Geometry: see drawing. Coordinates: mm, zero at the bounding-box minimum. A direction names the side the tool comes from. Round coordinates to 2 decimals unless told otherwise and drop trailing zeros. Write each loop counter-clockwise with the first axis right and the second up, starting at its lowest first coordinate (ties: lowest second). Pieces come first, ordered by that corner, then holes.
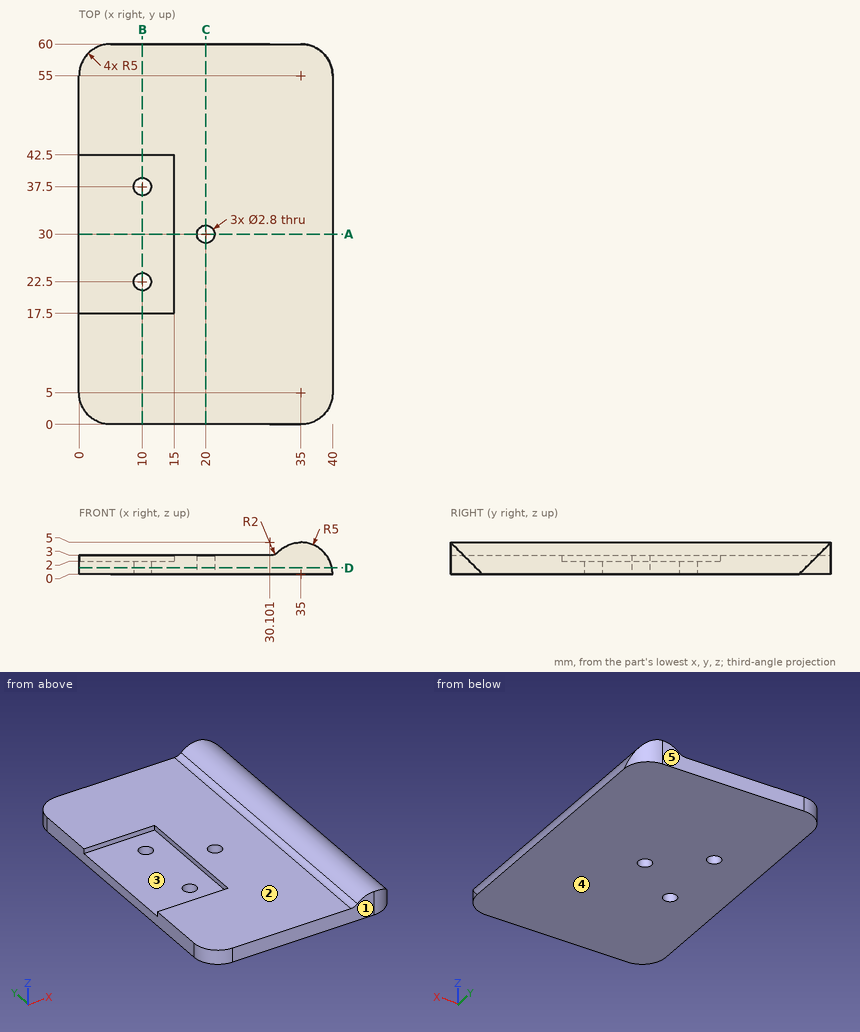
Q1. Set-up query: the marked faces 1 and 2. Return all of +Z, -Z, +X, -X, +Y, -Y with unobstructed straight access to the full face (end or side cutting, diameter ignored); none if empty.
Q2. Pin query (flat end, axial travel): P1, Ø2.5, axis at x = 20, y = 30, coming from the -Z side; P2, Ø8, axis at x = 16, y = 42.5, coming from the +Z side; P3, Ø0.8, axis at y = 28.5, z = 2.5, coming from the -X side; P4, Ø4.5, axis at x = 6.5, y = 27, coming from the +Z side. Return the tip coordinate at first contact, or that it passes through.
Q3. Section query A-A, the plane y = 30. Output: boundary loops of the cut face in (x, z).
Q4. Section query C-C, the plane x = 20. Output: boundary loops of the cut face in (y, z), and give its area (3 significant figures).
Q5. Mould query, pull axis Y, two halves, no side actions, for the marked faces 3, 4 and 5. Classes: pulls with the +Y half, pulls with the -Y half, needs draft (parallel to the pull), parting line crosses it, or undercut.
Q6. Line query: line 1 (Y direction, x = 10, z = 0.9); line 2 (Y direction, x = 20, z = 1.75); line 3 (Z direction, x = 20, y = 56). Output: solid intervals per line, ascending.
Q7. Section query D-D, the plane z = 1. Output: boundary loops of the cut face in (x, y).
Q8. Section query B-B, the plane x = 10. Output: boundary loops of the cut face in (y, z).
Filled in:
1. face 1: +Z, -Z, +X, -X, -Y
1. face 2: +Z, -X, +Y, -Y
2. P1: passes through
2. P2: stops at z = 3
2. P3: stops at x = 15
2. P4: stops at z = 2
3. outline: (0, 0) - (18.6, 0) - (18.6, 3) - (15, 3) - (15, 2) - (0, 2) - close; (21.4, 0) - (40, 0) arc R5 ccw to (31.5, 3.57) arc R2 cw to (30.1, 3) - (21.4, 3) - close
4. outline: (0, 0) - (28.6, 0) - (28.6, 3) - (0, 3) - close; (31.4, 0) - (60, 0) - (60, 3) - (31.4, 3) - close
4. area: 172 mm2
5. face 3: undercut
5. face 4: needs draft
5. face 5: pulls with the +Y half
6. line 1: y = 0 to 21.1, 23.9 to 36.1, 38.9 to 60
6. line 2: y = 0 to 28.6, 31.4 to 60
6. line 3: z = 0 to 3
7. outline: (0, 5) arc R5 ccw to (5, 0) - (35, 0) arc R5 ccw to (39.9, 4) - (39.9, 56) arc R5 ccw to (35, 60) - (5, 60) arc R5 ccw to (0, 55) - close; hole circle Ø2.8 at (10, 22.5); hole circle Ø2.8 at (10, 37.5); hole circle Ø2.8 at (20, 30)
8. outline: (0, 0) - (21.1, 0) - (21.1, 2) - (17.5, 2) - (17.5, 3) - (0, 3) - close; (23.9, 0) - (36.1, 0) - (36.1, 2) - (23.9, 2) - close; (38.9, 0) - (60, 0) - (60, 3) - (42.5, 3) - (42.5, 2) - (38.9, 2) - close
